Check sheet for the modelled part. Datum: model origin and axes. Units: mm. Face numbers are marked on the shaded views. A direction names the side the tool comes from. Round coordinates to 2 decimals unless told otherwise and drop trailing zeros. Order: outer loops, then holes, each group sorted by start corner. A loop starts at its lowest first (then second) coordinate and runs counter-clockwise, first axis right, second up. Notation, with made-up numbers: M 46,49 L 68,49 A12 cw 68,59 Z; hole C 42.25,66 d2. An arc over 180 degrees is marked long. One line per item, written item: value. Start each with the question number.
(1) Cross-section at B-B, the plane x = -15. Enter the section's corners in (y, z).
(2) Release check for a two-part mould opening along X. For the marked faces 1, 2, 3 and 4 record: released by +X, released by -X, zero draft, split by the parting line, or undercut.
(3) Access from +Z, -Z, +X, -X, +Y, -Y to the whole of each face (thin tool, end or side, straight path). Record for the marked faces 5, 6 and 7.
(4) Cross-section at C-C, the plane z = 6.5. Enter the section's corners in (x, y), and give its area (3 significant figures).
(5) Cross-section at D-D, the plane y = -9. Enter the section's corners in (x, z), and give its area (3 significant figures).
(6) Cross-section at A-A, the plane y = 0. Enter the section's corners in (x, z).
(7) Thickness scan on L1, parallel to X at y = 0, z = 7; L2, parallel to Y at x = 21.5, z = -15; L3, parallel to Y at x = 12, z = 3.5. Record the ranges inside material, lowest first.
(8) Depth check by flat-ended pin: pin 1 Ø16.5 at (x, z) = (8, -6) entering from +Y; pin 2 Ø8 at (x, z) = (12.5, 1) entering from +Y; pin 3 Ø4 at (x, y) = (6.5, -4.5) entering from -Z; pin 4 Ø1.5 at (x, z) = (-2.5, -5.5) entering from -Y. Enter the tip coordinate at first touch or a pass-through.
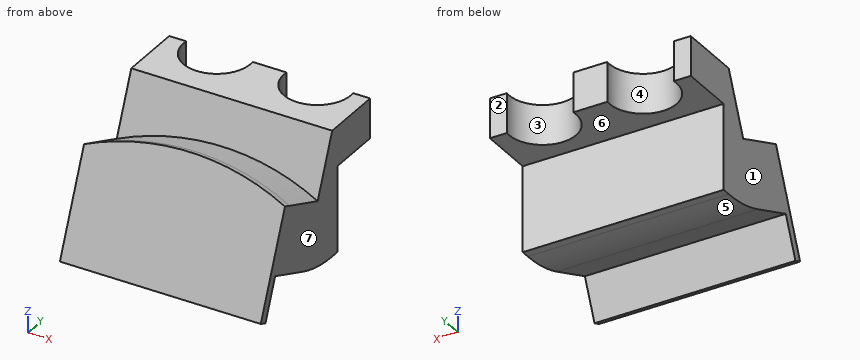
Autodesk Inventor part; units mm, degrees
ref_plane "YZ Plane" through (0, 0, 0) normal (1, 0, 0) x (0, 1, 0)
ref_plane "XZ Plane" through (0, 0, 0) normal (0, 1, 0) x (-1, 0, 0)
ref_plane "XY Plane" through (0, 0, 0) normal (0, 0, 1) x (1, 0, 0)
sketch "Sketch1" plane through (0, 0, 0) normal (0, 0, 1) x (1, 0, 0)
  arc A0 (-19.9373, 1) -> (-4.0627, 1) centre (-12, 0) ccw
  arc A1 (4.0627, 1) -> (19.9373, 1) centre (12, 0) ccw
  line L0 (0, 1) -> (-4.0627, 1)
  line L1 (0, 1) -> (4.0627, 1)
  line L2 (-24, 0) -> (-24, 1)
  line L3 (-19.9373, 1) -> (-24, 1)
  line L4 (24, 0) -> (24, 1)
  line L5 (24, 1) -> (19.9373, 1)
  line L6 (24, 0) -> (24, -12)
  line L7 (24, -12) -> (-24, -12)
  line L8 (-24, -12) -> (-24, 0)
  line L9 (24, 1) -> (24, -12)
  line L10 (24, -12) -> (-24, -12)
  line L11 (-24, -12) -> (-24, 1)
  line L12 (-24, 1) -> (-19.9373, 1)
  line L13 (-4.0627, 1) -> (4.0627, 1)
  line L14 (19.9373, 1) -> (24, 1)
  point P0 (0, 0)
  dimension "d4" = 12
  dimension "d5" = 12
  dimension "d6" = 1
  dimension "d7" = 12
extrude "Extrusion1" add sketch "Sketch1" along normal blind 9.5
sketch "Sketch2" plane through (-24, -12, 0) normal (0, -1, 0) x (1, 0, 0)
  line L0 (0, 9.5) -> (48, 9.5)
  line L1 (0, 9.5) -> (48, 9.5)
  line L2 (48, 9.5) -> (48, -20.5)
  line L3 (48, -20.5) -> (0, -20.5)
  line L4 (0, -20.5) -> (0, 9.5)
  point P0 (24, 0)
  dimension "d10" = 30
extrude "Extrusion2" add sketch "Sketch2" along normal blind 2
sketch "Sketch3" plane through (-24, -14, 0) normal (0, -1, 0) x (1, 0, 0)
  line L0 (48, 9.5) -> (0, 9.5)
  line L1 (0, 9.5) -> (0, -20.5)
  line L2 (0, -20.5) -> (48, -20.5)
  line L3 (48, -20.5) -> (48, 9.5)
  point P0 (24, 0)
revolve "Revolution1" add sketch "Sketch3" angle 22.5 about axis through (24, -14, 9.5) along (-1, 0, 0)
sketch "Sketch4" plane through (-24, -14, 9.5) normal (0, -0.9238795, 0.3826834) x (1, 0, 0)
  line L0 (48, -27.7164) -> (48, -30)
  line L1 (48, -30) -> (0, -30)
  line L2 (0, -30) -> (0, -15)
  line L3 (48, -15) -> (48, -30)
  line L4 (48, -8.0115) -> (48, -26.951)
  line L5 (0, -26.951) -> (0, -8.0115)
  arc A0 (48, -15) -> (0, -15) centre (24, -70.1) ccw
  point P0 (24, -3.4193)
extrude "Extrusion3" add sketch "Sketch4" along normal blind 12
sketch "Sketch5" plane through (-24, -25.0866, 14.0922) normal (0, -0.9238795, 0.3826834) x (1, 0, 0)
  arc A0 (48, -15) -> (0, -15) centre (24, -70.1) ccw
  arc A1 (48, -15) -> (0, -15) centre (24, -70.1) ccw
  line L0 (48, -15) -> (48, -40)
  line L1 (0, -15) -> (0, -40)
  line L2 (0, -40) -> (48, -40)
  point P0 (24, -3.4193)
  dimension "d19" = 25
  dimension "d20" = 25
extrude "Extrusion4" add sketch "Sketch5" along normal blind 2
properties part number "HatSensorMount03FB"
Values found:
1. outline: M -42.24,-22.1 L -40.39,-22.86 L -36.57,-13.62 L -25.48,-18.22 A30 ccw -14,-20.5 L -12,-20.5 L -12,0 L -7.42,0 L -7.42,9.5 L -14,9.5 L -18.55,-1.5 L -31.49,3.86 Z
2. face 1: released by -X
2. face 2: zero draft
2. face 3: undercut
2. face 4: undercut
3. face 5: -Z, +X, -X
3. face 6: -Z, +X, -X, +Y
3. face 7: +Z, -Z, +X, +Y, -Y
4. outline: M -24,-15.24 L 24,-15.24 L 24,1 L 19.94,1 A8 cw long 4.06,1 L -4.06,1 A8 cw long -19.94,1 L -24,1 Z
4. area: 547 mm^2
5. outline: M -24,0 L 24,0 L 24,9.5 L -24,9.5 Z
5. area: 456 mm^2
6. outline: M -24,0 L -20,0 L -20,9.5 L -24,9.5 Z; M -4,0 L 4,0 L 4,9.5 L -4,9.5 Z; M 20,0 L 24,0 L 24,9.5 L 20,9.5 Z
7. L1: -24 to -20, -4 to 4, 20 to 24
7. L2: -39.3 to -37.14, -33.25 to -12
7. L3: -31.64 to -28.81, -16.49 to -8
8. pin 1: y = 1
8. pin 2: y = -6.61
8. pin 3: z = 0
8. pin 4: y = -35.68
